```python
from build123d import *

# Parameters (mm, degrees)
CYLINDER1886_R               = 1.5
CYLINDER1886_DEPTH           = 20
CYLINDER1886_PLACEMENT_ANGLE = -112.5
CYLINDER1887_R               = 1.5
CYLINDER1887_DEPTH           = 20
CYLINDER1887_PLACEMENT_ANGLE = 112.5
CYLINDER1889_R               = 1.5
CYLINDER1889_DEPTH           = 20
CYLINDER1889_PLACEMENT_ANGLE = 112.5
CYLINDER1888_R               = 1.5
CYLINDER1888_DEPTH           = 20
CYLINDER1888_PLACEMENT_ANGLE = -112.5
BOX747_W                     = 16
BOX747_H                     = 19
BOX747_DEPTH                 = 3
BOX746_W                     = 26
BOX746_H                     = 37
BOX746_DEPTH                 = 3
CUT684_PLACEMENT_ANGLE       = 180


with BuildPart() as obj1:
    # Cylinder1886 → Cylinder1886 (new body)
    with BuildSketch(Plane.XY):
        Circle(CYLINDER1886_R)
    extrude(amount=CYLINDER1886_DEPTH)


with BuildPart() as obj1_1:
    # Cylinder1886 placement: moved
    add(obj1.part.moved(Location((-8, 34, 51))).rotate(Axis((-8, 34, 51), (0, 0, 1)), CYLINDER1886_PLACEMENT_ANGLE))


with BuildPart() as obj2:
    # Cylinder1887 → Cylinder1887 (new body)
    with BuildSketch(Plane.XY):
        Circle(CYLINDER1887_R)
    extrude(amount=CYLINDER1887_DEPTH)


with BuildPart() as obj2_1:
    # Cylinder1887 placement: moved
    add(obj2.part.moved(Location((8, 62, 51))).rotate(Axis((8, 62, 51), (0, 0, -1)), CYLINDER1887_PLACEMENT_ANGLE))


with BuildPart() as obj3:
    # Cylinder1889 → Cylinder1889 (new body)
    with BuildSketch(Plane.XY):
        Circle(CYLINDER1889_R)
    extrude(amount=CYLINDER1889_DEPTH)


with BuildPart() as obj3_1:
    # Cylinder1889 placement: moved
    add(obj3.part.moved(Location((-8, 62, 51))).rotate(Axis((-8, 62, 51), (0, 0, -1)), CYLINDER1889_PLACEMENT_ANGLE))


with BuildPart() as compound846:
    # Cylinder1888 → Cylinder1888 (new body)
    with BuildSketch(Plane.XY):
        Circle(CYLINDER1888_R)
    extrude(amount=CYLINDER1888_DEPTH)


with BuildPart() as compound846_1:
    # Cylinder1888 placement: moved
    add(compound846.part.moved(Location((8, 34, 51))).rotate(Axis((8, 34, 51), (0, 0, 1)), CYLINDER1888_PLACEMENT_ANGLE))

    # Compound846: union obj1, obj2, obj3
    add(obj1_1.part)
    add(obj2_1.part)
    add(obj3_1.part)


with BuildPart() as compound846_2:
    # Compound846 placement: moved
    add(compound846_1.part.moved(Location((0, -94, -180))))


with BuildPart() as krychle746:
    # Box747 → Box747 (new body)
    with BuildSketch(Plane(origin=(-8, 37, 27), x_dir=(1, 0, 0), z_dir=(0, 0, 1))):
        with Locations((8, 9.5)):
            Rectangle(BOX747_W, BOX747_H)
    extrude(amount=BOX747_DEPTH)


with BuildPart() as cut685:
    # Box746 → Box746 (new body)
    with BuildSketch(Plane(origin=(-13, 31, 27), x_dir=(1, 0, 0), z_dir=(0, 0, 1))):
        with Locations((13, 18.5)):
            Rectangle(BOX746_W, BOX746_H)
    extrude(amount=BOX746_DEPTH)

    # Cut684: cut Krychle746
    add(krychle746.part, mode=Mode.SUBTRACT)


with BuildPart() as cut685_1:
    # Cut684 placement: moved
    add(cut685.part.moved(Location((0, 2, -94))).rotate(Axis((0, 2, -94), (1, 0, 0)), CUT684_PLACEMENT_ANGLE))

    # Cut685: cut Compound846
    add(compound846_2.part, mode=Mode.SUBTRACT)


with BuildPart() as cut685_2:
    # Cut685 placement: moved
    add(cut685_1.part.moved(Location((0, 0, -3))))


solid = cut685_2.part
```
Read the model definition and answer for the solid it produces. Units are mm, in the model's axes. A direction names the side the tool comes from. Give positions to 0.01 mm unless a question says otherwise; leave off trailing zeros. Write each loop counter-clockwise with the first axis right and the second up, starting at its lowest first coordinate (ties: lowest second). Pieces come first, ordered by that corner, then holes. Notation, with made-up numbers: (48, 48) -> (71, 48) arc R7 cw to (71, 60) -> close; hole circle Ø6 at (40, -10). An arc over 180 degrees is marked (long way). Answer in a Markdown table with one row per item.
1) Determine the mould class of faces 1 (the flat face through (0, -56, -124)), 2 (the flat face through (13, -47, -125)), 3 (the cylindrical face through (7.869, -33.494, -125.521)) for opening direction X: released by +X, released by -X, zero draft, split by the parting line, or undercut.
Results list:
| item | result |
|---|---|
| face 1 | zero draft |
| face 2 | released by +X |
| face 3 | undercut |
2) Section B-B on y = -36 is taken. Give the vertices of the cut face in (x, z), plus the area to 3 significant figures.
Results list:
| item | result |
|---|---|
| outline | (-13, -127) -> (-8, -127) -> (-8, -124) -> (-13, -124) -> close; (8, -127) -> (13, -127) -> (13, -124) -> (8, -124) -> close |
| area | 30.0 mm^2 |
3) Section A-A on x = 4.75 is taken. Give the vertices of the cut face in (y, z).
Results list:
| item | result |
|---|---|
| outline | (-66, -127) -> (-54, -127) -> (-54, -124) -> (-66, -124) -> close; (-35, -127) -> (-29, -127) -> (-29, -124) -> (-35, -124) -> close |
4) Straight lines are drawn through the part: line 1 (X direction, y = -60, z = -124.65); line 2 (X direction, y = -37, z = -125.05); line 3 (Y direction, x = -7, z = -125.9). For each, find the intervals that lie inside material, in ascending order. Write a range as [from, to].
Results list:
| item | result |
|---|---|
| line 1 | [-13, -9.5], [-6.5, 6.5], [9.5, 13] |
| line 2 | [-13, -8], [8, 13] |
| line 3 | [-66, -61.12], [-58.88, -54], [-35, -33.12], [-30.88, -29] |
5) Section D-D on z = -125.35 is taken. Give the vertices of the cut face in (x, y).
Results list:
| item | result |
|---|---|
| outline | (-13, -66) -> (13, -66) -> (13, -29) -> (-13, -29) -> close; hole circle Ø3 at (-8, -60); hole circle Ø3 at (-8, -32); hole (-8, -54) -> (8, -54) -> (8, -35) -> (-8, -35) -> close; hole circle Ø3 at (8, -60); hole circle Ø3 at (8, -32) |
6) A tool of negligible diameter and unlimited length cuts with its end or side. For faces 4 (the flat face through (0, -35, -125)), 5 (the flat face through (0, -66, -125)), from which of +Z, -Z, +X, -X, +Y, -Y can it reach the whole face along a straight path? Write none if from no direction.
Results list:
| item | result |
|---|---|
| face 4 | +Z, -Z |
| face 5 | +Z, -Z, +X, -X, -Y |
7) Section C-C on y = -31.5 is taken. Give the vertices of the cut face in (x, z).
Results list:
| item | result |
|---|---|
| outline | (-13, -127) -> (-9.41, -127) -> (-9.41, -124) -> (-13, -124) -> close; (-6.59, -127) -> (6.59, -127) -> (6.59, -124) -> (-6.59, -124) -> close; (9.41, -127) -> (13, -127) -> (13, -124) -> (9.41, -124) -> close |
8) Each of these flat-tipped pins is pushed along its axis until it touches: pin 1 Ø5 at (x, y) = (8, -60) entering from -Z; pin 2 Ø1.8 at (x, y) = (-8, -32) entering from +Z. Where does it stop, or does it pass through?
Results list:
| item | result |
|---|---|
| pin 1 | z = -127 |
| pin 2 | through |
